Part model, mm, in its own coordinate system. A direction names the side the tool comes from. Coordinates: 2 decimals unless noted, no trailing zeros. Order: outer loops, then holes, each group sorted by start corner. A loop starts at its lowest first (then second) coordinate and runs counter-clockwise, first axis right, second up.
1) Pin check, flat tips, straight feed: pin 1 Ø5 at (y, z) = (13, 6) entering from +X; pin 2 Ø3 at (x, z) = (1, 5.5) entering from -Y; pin 3 Ø1.5 at (x, z) = (14, 4.5) entering from +Y. Stop position of each tip, or through.
2) Cut at C-C (x = 39.85). Give the number of separate pieces and of enclosed holes in the cut face, and give its area (3 significant figures).
3) Cut at A-A (y = 40.5). List the corners of the cut face in (x, z), and give its area (3 significant figures).
4) Mould opens along Y. For faces 5 (the cylindrical face through (-53.066, -49.259, 2.958)), 6 (the flat face through (-54.23, 58.01, 4.93)) say: +Y half, -Y half, draft (parallel to the pull), parting line (faces both ways), or undercut.
5) Wall check: L1, parallel to X at y = 39, z = 9.75; L2, parallel to X at y = -39, z = 2.5; L3, parallel to Y at x = 56.5, z = 3.5. Give the ranges that are in metal, low to high.
6) Cut at B-B (x = 10). List the corners of the cut face in (y, z), and give its area (3 significant figures).
7) Tool access for faces 1 (the flat face through (0, 6.149, 5)), 2 (the flat face through (63.15, -30.11, 4.93)), 3 (the cylindrical face through (36.2, -23.66, 7.97)), 4 (the flat face through (-62.665, 9.498, 4.93)): list every direction of +Z, -Z, +X, -X, +Y, -Y with a clear straight run to the whole face (end or side of a thin tool).
```python
from build123d import *

# Parameters (mm, degrees)
F0_R     = 4.6
F0_R_2   = 2.5
F1_DEPTH = 10
F0_R_3   = 3.6
F2_DEPTH = 6


# Not quite as in the source:
# - ends of sketch curves that miss each other by under 0.0002 mm in the source are joined


with BuildPart() as f1:
    # F0 (on Top) → F1 (new body)
    with BuildSketch(Plane.XY):
        with BuildLine():
            Line((-45.12993, 63.520274), (-63.589038, 52.344512))
            Line((-63.589038, 52.344512), (-64.491972, 51.645644))
            Line((-64.491972, 51.645644), (-65.195294, 50.763356))
            Line((-65.195294, 50.763356), (-65.706925, 49.675321))
            Line((-65.706925, 49.675321), (-66.018102, 48.35028))
            Line((-66.018102, 48.35028), (-69.517849, 23.448285))
            Line((-69.517849, 23.448285), (-69.565467, 22.06741))
            Line((-69.565467, 22.06741), (-69.321375, 20.551373))
            Line((-69.321375, 20.551373), (-68.771557, 18.920731))
            Line((-68.771557, 18.920731), (-67.92238, 17.202201))
            Line((-67.92238, 17.202201), (-66.786009, 15.407932))
            Line((-66.786009, 15.407932), (-58.427898, 3.420306))
            ThreePointArc((-58.427898, 3.420306), (-58.1136589115, 2.780672761), (-58.0056, 2.076258))
            Line((-58.0056, 2.076258), (-58.0056, -21.994915))
            ThreePointArc((-58.0056, -21.994915), (-58.1134934985, -22.6988030848), (-58.427266754, -23.3380571713))
            Line((-58.427266754, -23.3380571713), (-67.733177, -36.698447))
            Line((-67.733177, -36.698447), (-68.737483, -38.320327))
            Line((-68.737483, -38.320327), (-69.450198, -39.883875))
            Line((-69.450198, -39.883875), (-69.867581, -41.370908))
            Line((-69.867581, -41.370908), (-70, -42.7495))
            Line((-70, -42.7495), (-70, -60.5007))
            ThreePointArc((-70, -60.5007), (-69.01608381, -62.87608381), (-66.6407, -63.86))
            Line((-66.6407, -63.86), (-20.34613, -63.86))
            ThreePointArc((-20.34613, -63.86), (-19.5423824877, -63.718277595), (-18.8355788311, -63.3102042013))
            Line((-18.8355788311, -63.3102042013), (-5.655221, -52.25057))
            ThreePointArc((-5.655221, -52.25057), (-4.9484172103, -51.8424972951), (-4.14467, -51.700775))
            Line((-4.14467, -51.700775), (4.14467, -51.700775))
            ThreePointArc((4.14467, -51.700775), (4.9484172103, -51.8424972951), (5.6552206765, -52.2505703856))
            Line((5.6552206765, -52.2505703856), (18.835579, -63.310204))
            ThreePointArc((18.835579, -63.310204), (19.5423824877, -63.718277595), (20.34613, -63.86))
            Line((20.34613, -63.86), (66.64, -63.86))
            ThreePointArc((66.64, -63.86), (69.0158787848, -62.8758787848), (70, -60.5))
            Line((70, -60.5), (70, -42.7495))
            Line((70, -42.7495), (69.867655, -41.370921))
            Line((69.867655, -41.370921), (69.45051, -39.883911))
            Line((69.45051, -39.883911), (68.738189, -38.320362))
            Line((68.738189, -38.320362), (67.734411, -36.698447))
            Line((67.734411, -36.698447), (58.431323, -23.33483))
            ThreePointArc((58.431323, -23.33483), (58.1178034861, -22.6957823028), (58.01, -21.992181))
            Line((58.01, -21.992181), (58.01, 2.079652))
            ThreePointArc((58.01, 2.079652), (58.1179688317, 2.7837800001), (58.4319542472, 3.4232068277))
            Line((58.4319542472, 3.4232068277), (66.783488, 15.407932))
            Line((66.783488, 15.407932), (67.921136, 17.204755))
            Line((67.921136, 17.204755), (68.770985, 18.924136))
            Line((68.770985, 18.924136), (69.321132, 20.553655))
            Line((69.321132, 20.553655), (69.565833, 22.06785))
            Line((69.565833, 22.06785), (69.51871, 23.448285))
            Line((69.51871, 23.448285), (66.018963, 48.35028))
            Line((66.018963, 48.35028), (65.698808, 49.700863))
            Line((65.698808, 49.700863), (65.172247, 50.800958))
            Line((65.172247, 50.800958), (64.474805, 51.662632))
            Line((64.474805, 51.662632), (63.589037, 52.344512))
            Line((63.589037, 52.344512), (45.129929, 63.520274))
            ThreePointArc((45.129929, 63.520274), (44.5446477821, 63.7734755253), (43.912842, 63.86))
            Line((43.912842, 63.86), (20.34613, 63.86))
            ThreePointArc((20.34613, 63.86), (19.5423827897, 63.7182777049), (18.8355793235, 63.3102046144))
            Line((18.8355793235, 63.3102046144), (5.655221, 52.250571))
            ThreePointArc((5.655221, 52.250571), (4.9484175123, 51.842497405), (4.14467, 51.700775))
            Line((4.14467, 51.700775), (-4.14467, 51.700775))
            ThreePointArc((-4.14467, 51.700775), (-4.9484175123, 51.842497405), (-5.6552211689, 52.2505707987))
            Line((-5.6552211689, 52.2505707987), (-18.835579, 63.310205))
            ThreePointArc((-18.835579, 63.310205), (-19.5423827897, 63.7182777049), (-20.34613, 63.86))
            Line((-20.34613, 63.86), (-43.912843, 63.86))
            ThreePointArc((-43.912843, 63.86), (-44.5446487821, 63.7734755253), (-45.12993, 63.520274))
        make_face()
        with Locations((-56.5, -50.34)):
            Circle(F0_R, mode=Mode.SUBTRACT)
        with Locations((-39.85, -51.178)):
            Circle(F0_R, mode=Mode.SUBTRACT)
        with Locations((-39.85, -41.178)):
            Circle(F0_R_2, mode=Mode.SUBTRACT)
        with Locations((-39.85, -20.858)):
            Circle(F0_R, mode=Mode.SUBTRACT)
        with Locations((-39.85, -0.538)):
            Circle(F0_R_2, mode=Mode.SUBTRACT)
        with Locations((-10, -9.96)):
            Circle(F0_R, mode=Mode.SUBTRACT)
        with Locations((39.85, -51.178)):
            Circle(F0_R, mode=Mode.SUBTRACT)
        with Locations((56.5, -50.34)):
            Circle(F0_R, mode=Mode.SUBTRACT)
        with Locations((39.85, -41.178)):
            Circle(F0_R_2, mode=Mode.SUBTRACT)
        with Locations((10, -9.96)):
            Circle(F0_R, mode=Mode.SUBTRACT)
        with Locations((39.85, -20.858)):
            Circle(F0_R, mode=Mode.SUBTRACT)
        with Locations((39.85, -0.538)):
            Circle(F0_R_2, mode=Mode.SUBTRACT)
        with Locations((-39.85, 9.462)):
            Circle(F0_R, mode=Mode.SUBTRACT)
        with Locations((-56.5, 29.36)):
            Circle(F0_R, mode=Mode.SUBTRACT)
        with Locations((-31.925, 29.36)):
            Circle(F0_R_2, mode=Mode.SUBTRACT)
        with Locations((-39.85, 49.462)):
            Circle(F0_R, mode=Mode.SUBTRACT)
        with BuildLine():
            Line((-26.57, 37.54), (-26.57, 46.54))
            ThreePointArc((-26.57, 46.54), (-23.57, 49.54), (-20.57, 46.54))
            Line((-20.57, 46.54), (-20.57, 37.54))
            ThreePointArc((-20.57, 37.54), (-23.57, 34.54), (-26.57, 37.54))
        make_face(mode=Mode.SUBTRACT)
        with BuildLine():
            Line((-17.5, 15.199075), (-17.5, 21.099375))
            ThreePointArc((-17.5, 21.099375), (-14.8493603037, 27.4985853037), (-8.45015, 30.149225))
            Line((-8.45015, 30.149225), (8.45015, 30.149225))
            ThreePointArc((8.45015, 30.149225), (14.8493603037, 27.4985853037), (17.5, 21.099375))
            Line((17.5, 21.099375), (17.5, 15.199075))
            ThreePointArc((17.5, 15.199075), (14.8493603037, 8.7998646963), (8.45015, 6.149225))
            Line((8.45015, 6.149225), (-8.45015, 6.149225))
            ThreePointArc((-8.45015, 6.149225), (-14.8493603037, 8.7998646963), (-17.5, 15.199075))
        make_face(mode=Mode.SUBTRACT)
        with Locations((31.925, 29.36)):
            Circle(F0_R_2, mode=Mode.SUBTRACT)
        with Locations((39.85, 9.462)):
            Circle(F0_R, mode=Mode.SUBTRACT)
        with Locations((56.5, 29.36)):
            Circle(F0_R, mode=Mode.SUBTRACT)
        with BuildLine():
            Line((20.57, 37.54), (20.57, 46.54))
            ThreePointArc((20.57, 46.54), (23.57, 49.54), (26.57, 46.54))
            Line((26.57, 46.54), (26.57, 37.54))
            ThreePointArc((26.57, 37.54), (23.57, 34.54), (20.57, 37.54))
        make_face(mode=Mode.SUBTRACT)
        with Locations((39.85, 49.462)):
            Circle(F0_R, mode=Mode.SUBTRACT)
    extrude(amount=F1_DEPTH)

    # F0 (on Top) → F2 (join)
    with BuildSketch(Plane.XY):
        with Locations((-39.85, 9.462)):
            Circle(F0_R)
        with Locations((-39.85, 9.462)):
            Circle(F0_R_2, mode=Mode.SUBTRACT)
        with Locations((-39.85, -20.858)):
            Circle(F0_R)
        with Locations((-39.85, -20.858)):
            Circle(F0_R_2, mode=Mode.SUBTRACT)
        with Locations((-39.85, -51.178)):
            Circle(F0_R)
        with Locations((-39.85, -51.178)):
            Circle(F0_R_2, mode=Mode.SUBTRACT)
        with Locations((39.85, -20.858)):
            Circle(F0_R)
        with Locations((39.85, -20.858)):
            Circle(F0_R_3, mode=Mode.SUBTRACT)
        with Locations((39.85, -51.178)):
            Circle(F0_R)
        with Locations((39.85, -51.178)):
            Circle(F0_R_3, mode=Mode.SUBTRACT)
        with Locations((39.85, 9.462)):
            Circle(F0_R)
        with Locations((39.85, 9.462)):
            Circle(F0_R_3, mode=Mode.SUBTRACT)
        with Locations((-39.85, 49.462)):
            Circle(F0_R)
        with Locations((-39.85, 49.462)):
            Circle(F0_R_2, mode=Mode.SUBTRACT)
        with Locations((39.85, 49.462)):
            Circle(F0_R)
        with Locations((39.85, 49.462)):
            Circle(F0_R_3, mode=Mode.SUBTRACT)
        with Locations((-10, -9.96)):
            Circle(F0_R)
        with Locations((-10, -9.96)):
            Circle(F0_R_2, mode=Mode.SUBTRACT)
        with Locations((10, -9.96)):
            Circle(F0_R)
        with Locations((10, -9.96)):
            Circle(F0_R_2, mode=Mode.SUBTRACT)
        with Locations((-56.5, -50.34)):
            Circle(F0_R)
        with Locations((-56.5, -50.34)):
            Circle(F0_R_3, mode=Mode.SUBTRACT)
        with Locations((56.5, 29.36)):
            Circle(F0_R)
        with Locations((56.5, 29.36)):
            Circle(F0_R_2, mode=Mode.SUBTRACT)
        with Locations((56.5, -50.34)):
            Circle(F0_R)
        with Locations((56.5, -50.34)):
            Circle(F0_R_3, mode=Mode.SUBTRACT)
        with Locations((-56.5, 29.36)):
            Circle(F0_R)
        with Locations((-56.5, 29.36)):
            Circle(F0_R_2, mode=Mode.SUBTRACT)
    extrude(amount=F2_DEPTH)


solid = f1.part
```
Geometry check:
1. pin 1: stops at x = 66.84
1. pin 2: stops at y = -51.7
1. pin 3: stops at y = 59.88
2. separate pieces: 7
2. enclosed holes: 0
2. area: 857 mm2
3. outline: (-67.12, 0) - (-26.57, 0) - (-26.57, 10) - (-67.12, 10) - close; (-20.57, 0) - (20.57, 0) - (20.57, 10) - (-20.57, 10) - close; (26.57, 0) - (67.12, 0) - (67.12, 10) - (26.57, 10) - close
3. area: 1,220 mm2
4. face 5: undercut
4. face 6: +Y half
5. L1: x = -67.33 to -26.57, -20.57 to 20.57, 26.57 to 67.33
5. L2: x = -69.05 to -41.08, -38.62 to 38.62, 41.08 to 69.05
5. L3: y = -63.86 to -53.94, -46.74 to 26.86, 31.86 to 56.64
6. outline: (-55.9, 0) - (-12.46, 0) - (-12.46, 6) - (-14.56, 6) - (-14.56, 10) - (-55.9, 10) - close; (-7.46, 0) - (6.28, 0) - (6.28, 10) - (-5.36, 10) - (-5.36, 6) - (-7.46, 6) - close; (30.02, 0) - (55.9, 0) - (55.9, 10) - (30.02, 10) - close
6. area: 814 mm2
7. face 1: +Z, -Z
7. face 2: +Z, -Z, +X
7. face 3: +Z
7. face 4: +Z, -Z, -X
